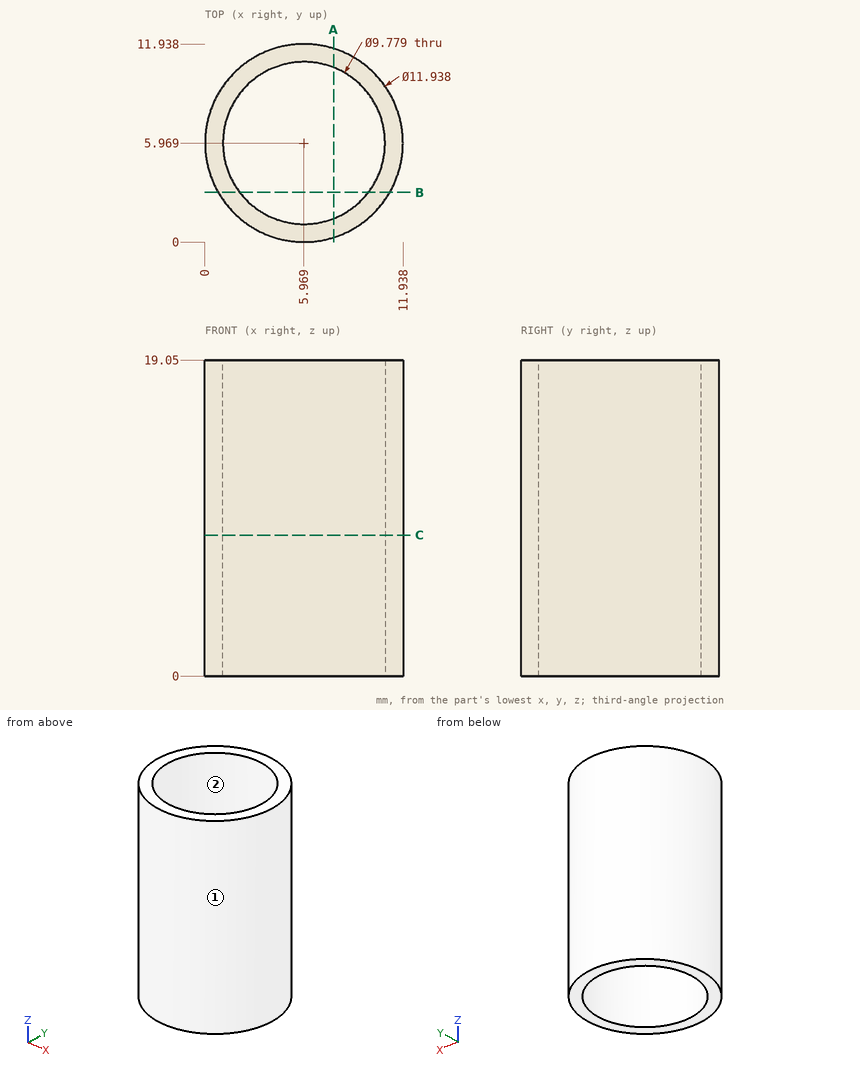
Can you work these out from the drawing? Everything is in mm from the part's minimum corner. Give positions to 0.01 mm unless a question says otherwise; leave off trailing zeros. Order: outer loops, then holes, each group sorted by start corner. A loop starts at its lowest first (then second) coordinate and runs counter-clockwise, first axis right, second up. Notation, with made-up numbers: M -25.75,-3 L -9.75,-3 A28 cw -9.75,30 Z; hole C 77,-35 d8. An arc over 180 degrees is marked long. Use a Markdown table: item, result. Add a question column.
1. If we mould it in two halves opening along Y, with no side actions, what happens to the marked faces 1 and 2? For each: +Y half, -Y half, draft (parallel to the pull), parting line (faces both ways), or undercut.
2. I need wall thicknesses on probe 1 along Y at (x, z) = (2.75, 4.25); probe 2 along X at (y, z) = (6.25, 16.75); probe 3 along Y at (x, z) = (8.5, 16.75). Which ranges of each line are inside material? Lowest first, please. Write a range as from..to.
3. For pin 1 Ø4 at (x, z) = (2.5, 9) entering from +Y; pin 2 Ø4 at (y, z) = (2.5, 7) entering from +X; pin 3 Ø5 at (y, z) = (10, 12) entering from +X, each with a flat end and sliding along its axis, tell me the tip position at first contact or that it passes through.
4. Suppose I cut it at B-B (y = 3). List the corners of the cut face in (x, z) for me.
5. Suppose I cut it at C-C (z = 8.5). List the corners of the cut face in (x, y) for me.
6. Suppose I cut it at A-A (x = 7.75). List the corners of the cut face in (y, z) for me, and give its area (3 significant figures).
Results list:
| question | item | result |
|---|---|---|
| 1 | face 1 | parting line |
| 1 | face 2 | undercut |
| 2 | probe 1 | y = 0.94..2.29, 9.65..11 |
| 2 | probe 2 | x = 0.01..1.09, 10.85..11.93 |
| 2 | probe 3 | y = 0.56..1.79, 10.15..11.37 |
| 3 | pin 1 | stops at y = 11.75 |
| 3 | pin 2 | stops at x = 11.75 |
| 3 | pin 3 | stops at x = 11.74 |
| 4 | outline | M 0.79,0 L 2.08,0 L 2.08,19.05 L 0.79,19.05 Z; M 9.85,0 L 11.15,0 L 11.15,19.05 L 9.85,19.05 Z |
| 5 | outline | C 5.97,5.97 d11.94; hole C 5.97,5.97 d9.78 |
| 6 | outline | M 0.27,0 L 1.42,0 L 1.42,19.05 L 0.27,19.05 Z; M 10.52,0 L 11.67,0 L 11.67,19.05 L 10.52,19.05 Z |
| 6 | area | 43.6 mm² |
